Verification items for the finished model (mm, model axes). A direction names the side the tool comes from. Round coordinates to 2 decimals unless told otherwise and drop trailing zeros. Write each loop counter-clockwise with the first axis right and the second up, starting at its lowest first coordinate (ties: lowest second). Pieces come first, ordered by that corner, then holes. Notation, with made-up numbers: (41.25, 76.5) -> (81.25, 76.5) arc R18 cw to (81.25, 92.5) -> close; hole circle Ø5 at (18, 57). An arc over 180 degrees is marked (long way). Answer as a JSON object with one key per item and string values. Group by question number.
(1) Set-up check for faces 4 (the face through (-12.795, 22.446, -24.52)), 5 (the face through (-12.468, -21.506, -20.879)), 6 (the face through (-18, 31, -38.1)): record each of +Z, -Z, +X, -X, +Y, -Y from which the full face is reachable in a straight line by a thin tool's end or side.
(2) Sectioned sample at D-D on z = -33.5. Record the cut outline in (x, y).
(3) Sectioned sample at A-A on z = -11. Count the separate pieces of the cut face and the enclosed holes in it, and give its area (3 significant figures).
(4) Draft check along Y on faces 1 (the face through (19, 12.7, -23)), 2 (the face through (-18, -31, -38.1)), 3 (the face through (-20.606, -10.29, -23.017)). Enter one of: released by +Y, released by -Y, zero draft, split by the parting line, or undercut.
(5) Gauge pin test, flat ends, axial feed: pin 1 Ø9.5 at (x, z) = (20, -14.5) entering from +Y; pin 2 Ø1 at (x, y) = (-3.5, 25) entering from -Z; pin 3 Ø15.5 at (x, z) = (26, -22.5) entering from -Y; pin 4 Ø1 at (y, z) = (23, -6) entering from -X. Record the tip position at first contact, or that the pin passes through.
(6) Sectioned sample at B-B on y = 31. Record the cut outline in (x, z).
(7) Scan lines: L1, parallel to Y at x = -19.5, z = -33.5 (3 decimals); L2, parallel to Y at x = 14.5, z = -34; L3, parallel to Y at x = -21.5, z = -29. Record each from-to range of solid material in increasing order. Write a range as from..to.
(8) Sectioned sample at C-C on x = 27.5. Record the cut outline in (y, z).
```python
from build123d import *

# Parameters (mm, degrees)
F1_DEPTH        = 12.7
F3_COUNT        = 3
F4_T            = 2.54
F4_T3_DEPTH     = 31.9573897847
F5_W            = 6.35
F5_H            = 21.5367313986
F5_R            = 1.651
F6_DEPTH        = 2.54
F6_COPIES_COUNT = 3


# Not quite as in the source:
# - a pattern or mirror of a feature is missing from the dataset's text; its kind, count and spacing are read off the source's solid
# - a shell that OpenCascade refuses in one call is made with other operations: the cavity is built on its own and cut out


with BuildPart() as f1:
    # F0 (on Front) → F1 (new body, symmetric)
    with BuildSketch(Plane.XZ):
        Polygon((11.7683534, 0), (0, 0), (0, -16.4057110057), (15.1905046899, -38.1), (38.4462606058, -38.1), align=None)
    extrude(amount=F1_DEPTH, both=True)

    # F3: F1 ×3 about axis
    f3_axis = Axis((0, 0, -8.2028555029), (0, 0, -1))


with BuildPart() as f1_1:
    add(f1.part)
    for i in range(1, F3_COUNT):
        add(f1.part.rotate(f3_axis, i * 360 / F3_COUNT))

    # F4: shell of thickness 2.54, made by hand


with BuildPart() as f4_core1:
    # F4_t2: copy of F1
    add(f1_1.part)

    # the walls: a layer under each face that stays
    f4_faces = [f4_core1.faces().sort_by_distance(p)[0] for p in [
        (-2.557172964, 0, 0),
        (22.8893045122, -12.7, -19.05),
        (-0.4461296281, -26.1727191826, -19.05),
        (-12.5536535014, -21.7435656851, -19.05),
        (-22.4431748842, -13.4727191826, -19.05),
        (22.8893045122, 12.7, -19.05),
        (25.1073070029, 0, -19.05),
        (-22.4431748842, 13.4727191826, -19.05),
        (-0.4461296281, 26.1727191826, -19.05),
        (-12.5536535014, 21.7435656851, -19.05),
    ]]
    thicken(f4_faces, amount=-F4_T, mode=Mode.SUBTRACT)

    # F4_s4 → F4_t3 (cut)
    with BuildSketch(Plane.XY.offset(-29.4173897847)):
        Polygon((7.354345464, -12.7381), (7.3323484187, -10.16), (5.865878735, -10.16), (5.1326438931, -11.43), align=None)
        Polygon((-14.7086909279, 0), (-12.4649923118, -1.27), (-11.7317574699, 0), (-12.4649923118, 1.27), align=None)
        Polygon((7.354345464, 12.7381), (7.3323484187, 10.16), (5.865878735, 10.16), (5.1326438931, 11.43), align=None)
    extrude(amount=F4_T3_DEPTH, mode=Mode.SUBTRACT)


with BuildPart() as f1_2:
    add(f1_1.part)

    # what is left inside the walls is the cavity
    f4_cavity = [f4_core1.part.solids().sort_by_distance(p)[0] for p in [
        (22.874997, 3.386667, -20.334569),
    ]]
    add(f4_cavity, mode=Mode.SUBTRACT)

    # F5 (on face) → F6 (cut)
    with BuildSketch(Plane(origin=(7.8966836583, 0, 5.5293174244), x_dir=(0, 1, 0), z_dir=(0.8191520443, 0, 0.5735764364))):
        with Locations((0, -20.5930502049)):
            Rectangle(F5_W, F5_H)
        with Locations((6.7175144213, -27.3105646262)):
            Circle(F5_R)
        with Locations((-6.7175144213, -13.8755357836)):
            Circle(F5_R)
    f6 = extrude(amount=-F6_DEPTH, mode=Mode.SUBTRACT)

    # F6_copies: F6 ×3 about axis
    f6_copies_axis = Axis((0, 0, 0), (0, 0, 1))
    for i in range(1, F6_COPIES_COUNT):
        add(f6.rotate(f6_copies_axis, i * 360 / F6_COPIES_COUNT), mode=Mode.SUBTRACT)


solid = f1_2.part
```
Computed values:
{
 "1": {"face 4": "-Z", "face 5": "+Z", "face 6": "-Z, +X, -X, +Y, -Y"},
 "2": {"outline": "(-28.61, -24.16) -> (-6.61, -36.86) -> (5.01, -16.72) -> (2.81, -15.45) -> (-7.26, -32.9) -> (-24.86, -22.74) -> (-14.78, -5.29) -> (-16.98, -4.02) -> close; (-28.61, 24.16) -> (-16.98, 4.02) -> (-14.78, 5.29) -> (-24.86, 22.74) -> (-7.26, 32.9) -> (2.81, 15.45) -> (5.01, 16.72) -> (-6.61, 36.86) -> close; (11.97, -12.7) -> (35.23, -12.7) -> (35.23, 12.7) -> (11.97, 12.7) -> (11.97, 10.16) -> (32.12, 10.16) -> (32.12, -10.16) -> (11.97, -10.16) -> close"},
 "3": {"separate pieces": "3", "enclosed holes": "0", "area": "326 mm2"},
 "4": {"face 1": "released by +Y", "face 2": "zero draft", "face 3": "undercut"},
 "5": {"pin 1": "y = 12.7", "pin 2": "z = -21.76", "pin 3": "y = -12.7", "pin 4": "through"},
 "6": {"outline": "(-23.2, -38.1) -> (-17, -38.1) -> (-6.17, -30.37) -> (-6.17, -38.1) -> (-3.23, -38.1) -> (-3.23, -23.84) -> close"},
 "7": {"L1": "-29.416..-25.836, -13.455..-8.375, 8.375..13.455, 25.836..29.416", "L2": "-12.7..-10.16, 10.16..12.7", "L3": "-24.62..-21.04, -16.92..-11.84, 11.84..16.92, 21.04..24.62"},
 "8": {"outline": "(-12.7, -38.1) -> (-10.16, -38.1) -> (-10.16, -26.9) -> (10.16, -26.9) -> (10.16, -38.1) -> (12.7, -38.1) -> (12.7, -22.47) -> (-12.7, -22.47) -> close"}
}
